from build123d import *

# Parameters (mm, degrees)
SKETCH3_W           = 73
SKETCH3_H           = 73
BOSS_EXTRUDE3_DEPTH = 10
SKETCH3_3_W         = 50.2
SKETCH3_3_H         = 50.2
CUT_EXTRUDE2_DEPTH  = 2
SKETCH4_R           = 2.925
CUT_EXTRUDE3_DEPTH  = 4
SKETCH13_R          = 1.75
CUT_EXTRUDE6_DEPTH  = 10
SKETCH5_W           = 44.2
SKETCH5_H           = 44.2
CUT_EXTRUDE4_DEPTH  = 1
SKETCH7_W           = 73
SKETCH7_H           = 73
SKETCH7_W_2         = 52.2
SKETCH7_H_2         = 52.2
BOSS_EXTRUDE5_DEPTH = 9.5
SKETCH8_W           = 10.7
SKETCH8_H           = 2.6
BOSS_EXTRUDE6_DEPTH = 14
FILLET1_R           = 0.25
SKETCH9_R           = 17.5
CUT_EXTRUDE5_DEPTH  = 10
BOSS_EXTRUDE7_DEPTH = 10
FILLET2_R           = 5
FILLET2_R_2         = 2
SKETCH15_W          = 73
SKETCH15_H          = 73
REBAIX_DEPTH        = 2
CUT_EXTRUDE11_START = -15.5
CUT_EXTRUDE11_DEPTH = 15.5
SKETCH19_R          = 1.6
CUT_EXTRUDE12_DEPTH = 85.84323793
CHAMFER1_SIZE       = 1.5


with BuildPart() as part:
    # Sketch3 → Boss-Extrude3 (new body)
    with BuildSketch(Plane(origin=(0, 0, 0), x_dir=(1, 0, 0), z_dir=(0, 1, 0))):
        Rectangle(SKETCH3_W, SKETCH3_H)
    extrude(amount=-BOSS_EXTRUDE3_DEPTH)

    # Sketch3<3> → Cut-Extrude2 (cut)
    with BuildSketch(Plane(origin=(0, 0, 0), x_dir=(1, 0, 0), z_dir=(0, 1, 0))):
        Rectangle(SKETCH3_3_W, SKETCH3_3_H)
    extrude(amount=-CUT_EXTRUDE2_DEPTH, mode=Mode.SUBTRACT)

    # Sketch4 → Cut-Extrude3 (cut)
    with BuildSketch(Plane(origin=(0, -2, 0), x_dir=(1, 0, 0), z_dir=(0, 1, 0))):
        with Locations(Location((-16.5, 16.5, 0), (0, 0, 270))):
            Circle(SKETCH4_R)
        with Locations(Location((16.5, 16.5, 0), (0, 0, 270))):
            Circle(SKETCH4_R)
        with Locations(Location((-16.5, -16.5, 0), (0, 0, 270))):
            Circle(SKETCH4_R)
        with Locations(Location((16.5, -16.5, 0), (0, 0, 270))):
            Circle(SKETCH4_R)
    extrude(amount=-CUT_EXTRUDE3_DEPTH, mode=Mode.SUBTRACT)

    # Sketch13 → Cut-Extrude6 (cut)
    with BuildSketch(Plane(origin=(0, -6, 0), x_dir=(1, 0, 0), z_dir=(0, 1, 0))):
        with Locations(Location((16.5, 16.5, 0), (0, 0, 270))):
            Circle(SKETCH13_R)
        with Locations(Location((16.5, -16.5, 0), (0, 0, 270))):
            Circle(SKETCH13_R)
        with Locations(Location((-16.5, -16.5, 0), (0, 0, 270))):
            Circle(SKETCH13_R)
        with Locations(Location((-16.5, 16.5, 0), (0, 0, 270))):
            Circle(SKETCH13_R)
    extrude(amount=-CUT_EXTRUDE6_DEPTH, mode=Mode.SUBTRACT)

    # Sketch5 → Cut-Extrude4 (cut)
    with BuildSketch(Plane(origin=(0, -2, 0), x_dir=(1, 0, 0), z_dir=(0, 1, 0))):
        Rectangle(SKETCH5_W, SKETCH5_H)
    extrude(amount=-CUT_EXTRUDE4_DEPTH, mode=Mode.SUBTRACT)

    # Sketch7 → Boss-Extrude5 (add)
    with BuildSketch(Plane(origin=(0, -2, 0), x_dir=(1, 0, 0), z_dir=(0, 1, 0))):
        Rectangle(SKETCH7_W, SKETCH7_H)
        Rectangle(SKETCH7_W_2, SKETCH7_H_2, mode=Mode.SUBTRACT)
    extrude(amount=BOSS_EXTRUDE5_DEPTH)

    # Sketch8 → Boss-Extrude6 (add)
    with BuildSketch(Plane(origin=(0, 7.5, 0), x_dir=(1, 0, 0), z_dir=(0, 1, 0))):
        with Locations((-23.85, 32.8)):
            Rectangle(SKETCH8_W, SKETCH8_H)
        with Locations((-23.85, -32.8)):
            Rectangle(SKETCH8_W, SKETCH8_H)
        with Locations((23.85, 32.8)):
            Rectangle(SKETCH8_W, SKETCH8_H)
        with Locations((23.85, -32.8)):
            Rectangle(SKETCH8_W, SKETCH8_H)
    extrude(amount=BOSS_EXTRUDE6_DEPTH)

    # Fillet1
    fillet1_edges = [part.edges().sort_by_distance(p)[0] for p in [
        (-36.5, 7.5, 0),
        (0, 7.5, 36.5),
        (36.5, 7.5, 0),
        (0, 7.5, -36.5),
    ]]
    fillet(fillet1_edges, radius=FILLET1_R)

    # Sketch9 → Cut-Extrude5 (cut)
    with BuildSketch(Plane(origin=(0, -3, 0), x_dir=(1, 0, 0), z_dir=(0, 1, 0))):
        with Locations(Location((0, 0, 0), (0, 0, 270))):
            Circle(SKETCH9_R)
    extrude(amount=-CUT_EXTRUDE5_DEPTH, mode=Mode.SUBTRACT)

    # Sketch10 → Boss-Extrude7 (add, symmetric)
    with BuildSketch(Plane(origin=(0, 0, 0), x_dir=(0, 0, -1), z_dir=(1, 0, 0))):
        Polygon((-36.5, -2), (-36.5, 4), (-38.25, 4), (-38.25, 20.375), (-56.25, 20.375), (-56.25, 15.375), (-41.25, 15.375), (-41.25, -2), align=None)
    extrude(amount=BOSS_EXTRUDE7_DEPTH, both=True)

    # Fillet2
    # the kernel refuses this fillet: 5, 2 mm, written as the material it adds along each edge
    with BuildSketch(Plane(origin=(-10, 4, 38.25), x_dir=(0, 0, -1), z_dir=(1, 0, 0))) as fillet2_piece_1:
        with BuildLine():
            CenterArc((5, 3.799671038), FILLET2_R, 180, 49.458398126)
            Line((0, 3.799671038), (0, 0))
            Line((0, 0), (1.75, 0))
        make_face()
    extrude(amount=20)
    # the kernel refuses this fillet: 5, 2 mm, written as the material it takes off along each edge
    with BuildSketch(Plane(origin=(-15, 20.375, 56.25), x_dir=(0, 0, -1), z_dir=(1, 0, 0)), Plane(origin=(-15, 20.375, 38.25), x_dir=(0, -1, 0), z_dir=(1, 0, 0))) as fillet2_2_piece_1:
        with BuildLine():
            CenterArc((FILLET2_R_2, -FILLET2_R_2), FILLET2_R_2, 90, 90)
            Line((0, -FILLET2_R_2), (0, 0))
            Line((0, 0), (FILLET2_R_2, 0))
        make_face()
    extrude(amount=30, mode=Mode.SUBTRACT)

    # CirPattern1: read off the stored shape, not the designer's step
    # CirPattern1: loft between two sections, ruled curve by curve
    cirpattern1_from = [
        Edge.make_three_point_arc((-38.25, 7.799671038, -10), (-37.791475531, 5.708020972, -10), (-36.5, 4, -10)),
        Edge.make_three_point_arc((-40.25, 20.375, -10), (-38.835786438, 19.789213562, -10), (-38.25, 18.375, -10)),
        Edge.make_three_point_arc((-56.25, 18.375, -10), (-55.664213562, 19.789213562, -10), (-54.25, 20.375, -10)),
        Edge.make_line((-41.25, -2, -10), (-36.5, -2, -10)),
        Edge.make_line((-40.25, 20.375, -10), (-54.25, 20.375, -10)),
        Edge.make_line((-56.25, 15.375, -10), (-41.25, 15.375, -10)),
        Edge.make_line((-41.25, 15.375, -10), (-41.25, -2, -10)),
        Edge.make_line((-38.25, 7.799671038, -10), (-38.25, 18.375, -10)),
        Edge.make_line((-56.25, 18.375, -10), (-56.25, 15.375, -10)),
        Edge.make_line((-36.5, -2, -10), (-36.5, 4, -10)),
    ]
    cirpattern1_to = [
        Edge.make_three_point_arc((-38.25, 7.799671038, 10), (-37.791475531, 5.708020972, 10), (-36.5, 4, 10)),
        Edge.make_three_point_arc((-40.25, 20.375, 10), (-38.835786438, 19.789213562, 10), (-38.25, 18.375, 10)),
        Edge.make_three_point_arc((-56.25, 18.375, 10), (-55.664213562, 19.789213562, 10), (-54.25, 20.375, 10)),
        Edge.make_line((-41.25, -2, 10), (-36.5, -2, 10)),
        Edge.make_line((-40.25, 20.375, 10), (-54.25, 20.375, 10)),
        Edge.make_line((-56.25, 15.375, 10), (-41.25, 15.375, 10)),
        Edge.make_line((-41.25, 15.375, 10), (-41.25, -2, 10)),
        Edge.make_line((-38.25, 7.799671038, 10), (-38.25, 18.375, 10)),
        Edge.make_line((-56.25, 18.375, 10), (-56.25, 15.375, 10)),
        Edge.make_line((-36.5, -2, 10), (-36.5, 4, 10)),
    ]
    cirpattern1 = Solid(Shell([*[Face.make_surface_from_curves(cirpattern1_from[k], cirpattern1_to[k]) for k in range(10)], Face(Wire(cirpattern1_from)), Face(Wire(cirpattern1_to))]))
    add(cirpattern1)

    # CirPattern1 2: loft between two sections, ruled curve by curve
    cirpattern1_2_from = [
        Edge.make_three_point_arc((10, 7.799671038, -38.25), (10, 5.708020972, -37.791475531), (10, 4, -36.5)),
        Edge.make_three_point_arc((10, 20.375, -40.25), (10, 19.789213562, -38.835786438), (10, 18.375, -38.25)),
        Edge.make_three_point_arc((10, 18.375, -56.25), (10, 19.789213562, -55.664213562), (10, 20.375, -54.25)),
        Edge.make_line((10, -2, -41.25), (10, -2, -36.5)),
        Edge.make_line((10, 20.375, -40.25), (10, 20.375, -54.25)),
        Edge.make_line((10, 15.375, -56.25), (10, 15.375, -41.25)),
        Edge.make_line((10, 15.375, -41.25), (10, -2, -41.25)),
        Edge.make_line((10, 7.799671038, -38.25), (10, 18.375, -38.25)),
        Edge.make_line((10, 18.375, -56.25), (10, 15.375, -56.25)),
        Edge.make_line((10, -2, -36.5), (10, 4, -36.5)),
    ]
    cirpattern1_2_to = [
        Edge.make_three_point_arc((-10, 7.799671038, -38.25), (-10, 5.708020972, -37.791475531), (-10, 4, -36.5)),
        Edge.make_three_point_arc((-10, 20.375, -40.25), (-10, 19.789213562, -38.835786438), (-10, 18.375, -38.25)),
        Edge.make_three_point_arc((-10, 18.375, -56.25), (-10, 19.789213562, -55.664213562), (-10, 20.375, -54.25)),
        Edge.make_line((-10, -2, -41.25), (-10, -2, -36.5)),
        Edge.make_line((-10, 20.375, -40.25), (-10, 20.375, -54.25)),
        Edge.make_line((-10, 15.375, -56.25), (-10, 15.375, -41.25)),
        Edge.make_line((-10, 15.375, -41.25), (-10, -2, -41.25)),
        Edge.make_line((-10, 7.799671038, -38.25), (-10, 18.375, -38.25)),
        Edge.make_line((-10, 18.375, -56.25), (-10, 15.375, -56.25)),
        Edge.make_line((-10, -2, -36.5), (-10, 4, -36.5)),
    ]
    cirpattern1_2 = Solid(Shell([*[Face.make_surface_from_curves(cirpattern1_2_from[k], cirpattern1_2_to[k]) for k in range(10)], Face(Wire(cirpattern1_2_from)), Face(Wire(cirpattern1_2_to))]))
    add(cirpattern1_2)

    # Sketch15 → rebaix (cut)
    with BuildSketch(Plane.XZ.offset(10)):
        Rectangle(SKETCH15_W, SKETCH15_H)
    extrude(amount=-REBAIX_DEPTH, mode=Mode.SUBTRACT)

    # Cut-Extrude11: read off the stored shape, not the designer's step
    # Cut-Extrude11 outline → Cut-Extrude11 (cut)
    with BuildSketch(Plane(origin=(0, 7.5, 0), x_dir=(1, 0, 0), z_dir=(0, 1, 0)).offset(CUT_EXTRUDE11_START)):
        with BuildLine():
            ThreePointArc((19.158528942, 6.947258634), (18.550604255, 0), (19.158528942, -6.947258634))
            ThreePointArc((19.158528942, -6.947258634), (25.181319297, -17.378426685), (36.500000379, -21.497981165))
            Line((36.500000379, -21.497981165), (36.500002527, 21.497981165))
            ThreePointArc((36.500002527, 21.497981165), (25.181320119, 17.378427376), (19.158528942, 6.947258634))
        make_face()
    extrude(amount=CUT_EXTRUDE11_DEPTH, mode=Mode.SUBTRACT)

    # Sketch19 → Cut-Extrude12 (cut, through all)
    with BuildSketch(Plane(origin=(0, -8, 0), x_dir=(-1, 0, 0), z_dir=(0, -1, 0))):
        with Locations(Location((0, -32.5, 0), (0, 0, 90))):
            Circle(SKETCH19_R)
        with Locations(Location((0, 32.5, 0), (0, 0, 90))):
            Circle(SKETCH19_R)
    extrude(amount=-CUT_EXTRUDE12_DEPTH, mode=Mode.SUBTRACT)

    # Chamfer1
    chamfer1_edges = [part.edges().sort_by_distance(p)[0] for p in [
        (16.5, -8, 14.75),
        (-16.5, -8, -18.25),
        (-16.5, -8, 14.75),
        (16.5, -8, -18.25),
    ]]
    chamfer(chamfer1_edges, length=CHAMFER1_SIZE)


solid = part.part
CAD build for the part. Positions are in the model's coordinates, mm. A direction names the side the tool comes from. Round coordinates to 2 decimals unless told otherwise and drop trailing zeros. Loops run counter-clockwise (first coordinate to the right, second up) from the corner with the lowest first, then second, coordinate; pieces in that order, holes last. Notation, with made-up numbers: (75.5, -14.5) - (100.5, -14.5) arc R25 ccw to (100.5, 12.5) - close; hole circle Ø1 at (50, 29.25). An arc over 180 degrees is marked (long way). Put each result on its own line as item: value.
1. 3-axis set-ups, long thin cutter, end or side, ignore diameter. For faces 1 (the flat face through (-18.5, 14, -33)), 2 (the flat face through (0, 15.375, 49)), 3 (the flat face through (24, 14, -31.5)): which of +Z, -Z, +X, -X, +Y, -Y reach the whole face in a straight line?
Geometry check:
face 1: +Z, -Z, +Y
face 2: +Z, +X, -X, -Y
face 3: +X, -X, +Y
2. Slice it at A-A on y = 13. Give the number of separate pieces and of enclosed holes in the cut face, and give its area (3 significant figures).
Geometry check:
separate pieces: 7
enclosed holes: 0
area: 291 mm²
3. Slice it at D-D on z = 42.5. List the corners of the cut face in (x, y) (3 decimals).
Geometry check:
outline: (-10, 15.375) - (10, 15.375) - (10, 20.375) - (-10, 20.375) - close
4. Slice it at B-B on z = -29.5. List the corners of the cut face in (x, y), and give its area (3 significant figures).
Geometry check:
outline: (-36.5, -8) - (36.5, -8) - (36.5, 7.25) arc R0.25 ccw to (36.25, 7.5) - (-36.25, 7.5) arc R0.25 ccw to (-36.5, 7.25) - close
area: 1,130 mm²
5. Two-plate mould, pull along Z, no slides. Class faces 4 (the flat face through (0, 7, 41.25)), 5 (the flat face through (-18, -6, -15)), 6 (the cylindrical face through (18.55, -5.54, -0.1)), 7 (the flat face through (0, -2, 39)): released by +Z, released by -Z, zero draft, split by the parting line, or undercut.
Geometry check:
face 4: released by +Z
face 5: undercut
face 6: undercut
face 7: zero draft
6. Wall check: line 1 (X direction, y = 4.5, z = 23.5); line 2 (X direction, y = 3.75, z = 32.5). Give the ranges that are in metal, low to high.
Geometry check:
line 1: -36.5 to -26.1, 26.1 to 36.5
line 2: -36.5 to -1.6, 1.6 to 36.5
7. Pin check, flat tips, straight feed: P1, Ø1.8, axis at x = -15.5, z = 17.5, coming from the +Y side; P2, Ø5, axis at y = 1, z = 45, coming from the -X side; P3, Ø8.5, axis at x = 23.5, y = 13, coming from the +Z side; P4, Ø1.6, axis at y = -1, z = -8, coming from the +X side. Stop position of each tip, or through.
Geometry check:
P1: y = -6
P2: through
P3: z = 34.1
P4: x = -25.1
